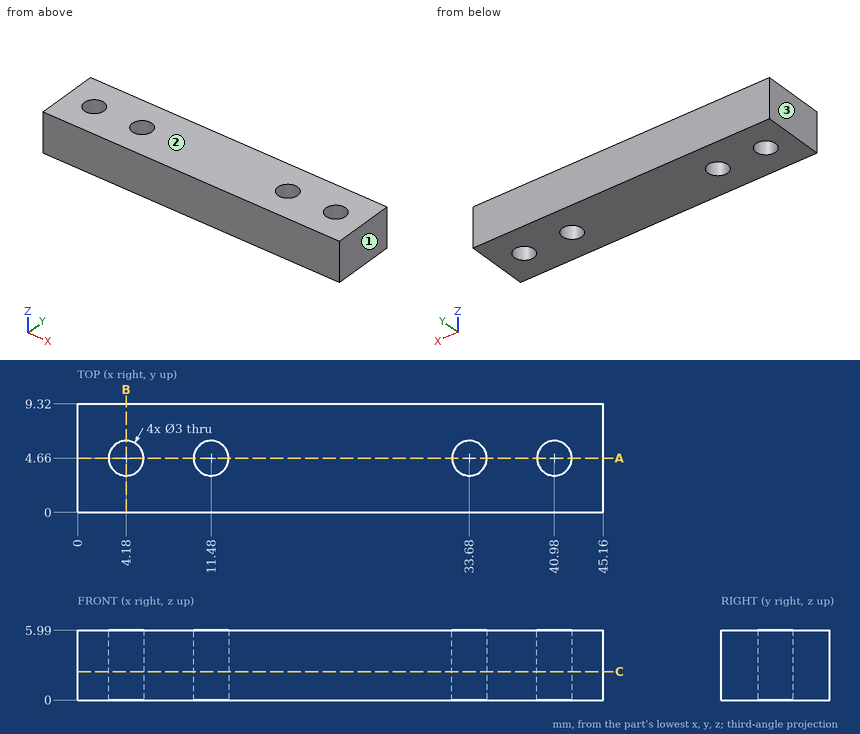
The drawing under review shows one solid part. Ordinate dimensions are in mm from its lowest x, y, z. Round coordinates to 2 decimals unless told otherwise and drop trailing zeros. Write each loop counter-clockwise with the first axis right and the second up, starting at its lowest first coordinate (ties: lowest second). Pieces come first, ordered by that corner, then holes.
(1) We need section B-B on x = 4.18. Give the boundary of the cut face in (y, z).
(2) We need section A-A on y = 4.66. Give the boundary of the cut face in (x, z), and give its area (3 significant figures).
(3) Mouldability with a two-part tool opening along X and no side actions: class the marked faces 1, 2 and 3 as +X half, -X half, draft (parallel to the pull), parting line (faces both ways), or undercut.
(4) Wall thickness on L1, parallel to X at y = 4.66, z = 4.8; L2, parallel to Y at x = 4.18, z = 4.2; L3, parallel to X at y = 4, z = 5.35: over which ranges is each line inside the solid? List them lowest first.
(5) We need section C-C on z = 2.45. Give the boundary of the cut face in (x, y), and give its area (3 significant figures).
Findings below:
1. outline: (0, 0) - (3.16, 0) - (3.16, 5.99) - (0, 5.99) - close; (6.16, 0) - (9.32, 0) - (9.32, 5.99) - (6.16, 5.99) - close
2. outline: (0, 0) - (2.68, 0) - (2.68, 5.99) - (0, 5.99) - close; (5.68, 0) - (9.98, 0) - (9.98, 5.99) - (5.68, 5.99) - close; (12.98, 0) - (32.18, 0) - (32.18, 5.99) - (12.98, 5.99) - close; (35.18, 0) - (39.48, 0) - (39.48, 5.99) - (35.18, 5.99) - close; (42.48, 0) - (45.16, 0) - (45.16, 5.99) - (42.48, 5.99) - close
2. area: 199 mm2
3. face 1: +X half
3. face 2: draft
3. face 3: -X half
4. L1: x = 0 to 2.68, 5.68 to 9.98, 12.98 to 32.18, 35.18 to 39.48, 42.48 to 45.16
4. L2: y = 0 to 3.16, 6.16 to 9.32
4. L3: x = 0 to 2.83, 5.53 to 10.13, 12.83 to 32.33, 35.03 to 39.63, 42.33 to 45.16
5. outline: (0, 0) - (45.16, 0) - (45.16, 9.32) - (0, 9.32) - close; hole circle Ø3 at (4.18, 4.66); hole circle Ø3 at (11.48, 4.66); hole circle Ø3 at (33.68, 4.66); hole circle Ø3 at (40.98, 4.66)
5. area: 393 mm2
